Could you check a few things on this model? Use its own coordinates, in mm. A direction names the side the tool comes from. Give positions to 0.01 mm unless a question says otherwise; leave off trailing zeros. Order: outer loops, then holes, each group sorted by start corner. A loop starts at its lowest first (then second) coordinate and runs counter-clockwise, first axis right, second up. Notation, with made-up numbers: (58, 64.25) - (78, 64.25) arc R24 cw to (78, 92.25) - close; hole circle Ø2 at (56.5, 34). An arc over 180 degrees is marked (long way). Put each result on its own line as item: value.
Autodesk Inventor part; units mm, degrees
ref_plane "YZ Plane" through (0, 0, 0) normal (1, 0, 0) x (0, 1, 0)
ref_plane "XZ Plane" through (0, 0, 0) normal (0, 1, 0) x (-1, 0, 0)
ref_plane "XY Plane" through (0, 0, 0) normal (0, 0, 1) x (1, 0, 0)
sketch "Sketch1" plane through (0, 0, 0) normal (0, 0, 1) x (1, 0, 0)
  line L0 (43, 15) -> (43, 0)
  line L1 (43, 0) -> (0, 0)
  line L2 (0, 0) -> (0, 110)
  line L3 (0, 110) -> (43, 110)
  line L4 (43, 110) -> (43, 95)
  line L5 (40.5, 15) -> (40.5, 2.5)
  line L6 (40.5, 2.5) -> (2.5, 2.5)
  line L7 (2.5, 2.5) -> (2.5, 107.5)
  line L8 (2.5, 107.5) -> (40.5, 107.5)
  line L9 (40.5, 107.5) -> (40.5, 95)
  line L10 (40.5, 95) -> (43, 95)
  line L11 (40.5, 15) -> (43, 15)
  dimension "d0" = 43
  dimension "d1" = 110
  dimension "d2" = 15
  dimension "d3" = 15
  dimension "d4" = 2.5
extrude "Extrusion1" add sketch "Sketch1" against normal blind 300
properties part number "c150x43x15x600"
1) Suppose I cut it at C-C, the plane z = -48. List the corners of the cut face in (x, y) for me.
Filled in:
outline: (0, 0) - (43, 0) - (43, 15) - (40.5, 15) - (40.5, 2.5) - (2.5, 2.5) - (2.5, 107.5) - (40.5, 107.5) - (40.5, 95) - (43, 95) - (43, 110) - (0, 110) - close
2) Suppose I cut it at B-B, the plane x = 22.5. List the corners of the cut face in (y, z) for me.
Filled in:
outline: (0, -300) - (2.5, -300) - (2.5, 0) - (0, 0) - close; (107.5, -300) - (110, -300) - (110, 0) - (107.5, 0) - close
3) Which directions (+Z, -Z, +X, -X, +Y, -Y) give clear straight access to the entire face, cutting with the end or side of a thin tool? Please do faces 1 (the flat face through (22, 0, -148)), 2 (the flat face through (22, 2.5, -148)).
Filled in:
face 1: +Z, -Z, +X, -X, -Y
face 2: +Z, -Z
4) If I drill on line 1 (X direction, y = 8.5, z = -256); line 2 (Y direction, x = 8.5, z = -283); line 3 (X direction, y = 43, z = -210), over which ranges is the centre line in solid material (lowest first)? Write a range as [from, to].
Filled in:
line 1: x = [0, 2.5], [40.5, 43]
line 2: y = [0, 2.5], [107.5, 110]
line 3: x = [0, 2.5]
5) Suppose I cut it at D-D, the plane y = 20.5. List the corners of the cut face in (x, z) for me.
Filled in:
outline: (0, -300) - (2.5, -300) - (2.5, 0) - (0, 0) - close
6) We'd pull the mould along X, two halves only. Please class faces 3 (the flat face through (21, 110, -148)), 4 (the flat face through (43, 8, -148)), 5 (the flat face through (40.5, 101, -148)): pulls with the +X half, pulls with the -X half, needs draft (parallel to the pull), parting line crosses it, or undercut.
Filled in:
face 3: needs draft
face 4: pulls with the +X half
face 5: undercut
7) Suppose I cut it at A-A, the plane y = 7.5. List the corners of the cut face in (x, z) for me.
Filled in:
outline: (0, -300) - (2.5, -300) - (2.5, 0) - (0, 0) - close; (40.5, -300) - (43, -300) - (43, 0) - (40.5, 0) - close
